```python
from build123d import *

# Parameters (mm, degrees)
SKETCH2_W                 = 304.8
SKETCH2_H                 = 101.6
SKETCH2_R                 = 6.35
SKETCH2_R_2               = 7
BOSS_EXTRUDE1_DEPTH       = 20
SKETCH3_R                 = 3.25
CUT_EXTRUDE1_DEPTH        = 162.883909021
CIRPATTERN1_COUNT         = 4
LPATTERN1_COUNT           = 2
LPATTERN1_PITCH           = 152.4
LPATTERN1_COPY_1_SKETCH_R = 3.25
LPATTERN1_COPY_1_DEPTH    = 162.883909021
LPATTERN1_COPY_2_SKETCH_R = 3.25
LPATTERN1_COPY_2_DEPTH    = 162.883909021
LPATTERN1_COPY_3_SKETCH_R = 3.25
LPATTERN1_COPY_3_DEPTH    = 162.883909021
SKETCH4_W                 = 35.387760229
SKETCH4_H                 = 49.864571232
CUT_EXTRUDE2_DEPTH        = 5


with BuildPart() as part:
    # Sketch2 → Boss-Extrude1 (new body)
    with BuildSketch(Plane(origin=(0, 0, 0), x_dir=(1, 0, 0), z_dir=(0, 1, 0))):
        Rectangle(SKETCH2_W, SKETCH2_H)
        with Locations(Location((0, 0, 0), (0, 0, 270))):
            Circle(SKETCH2_R, mode=Mode.SUBTRACT)
        with Locations(Location((-76.2, 0, 0), (0, 0, 270))):
            Circle(SKETCH2_R_2, mode=Mode.SUBTRACT)
        with Locations(Location((76.2, 0, 0), (0, 0, 270))):
            Circle(SKETCH2_R_2, mode=Mode.SUBTRACT)
    extrude(amount=BOSS_EXTRUDE1_DEPTH)

    # Sketch3 → Cut-Extrude1 (cut, through all)
    with BuildSketch(Plane(origin=(0, 20, 0), x_dir=(1, 0, 0), z_dir=(0, 1, 0))):
        with Locations(Location((-76.2, 19, 0), (0, 0, 270))):
            Circle(SKETCH3_R)
    cut_extrude1 = extrude(amount=-CUT_EXTRUDE1_DEPTH, mode=Mode.SUBTRACT)

    # CirPattern1: Cut-Extrude1 ×4 about axis
    cirpattern1_axis = Axis((-76.2, 0, 0), (0, 1, 0))
    for i in range(1, CIRPATTERN1_COUNT):
        add(cut_extrude1.rotate(cirpattern1_axis, i * 360 / CIRPATTERN1_COUNT), mode=Mode.SUBTRACT)

    # LPattern1: Cut-Extrude1 ×2
    with Locations(*[(i * LPATTERN1_PITCH, 0, 0) for i in range(1, LPATTERN1_COUNT)]):
        add(cut_extrude1, mode=Mode.SUBTRACT)

    # LPattern1 copy 1 sketch → LPattern1 copy 1 (cut, through all)
    with BuildSketch(Plane(origin=(76.2, 20, -76.2), x_dir=(0, 0, -1), z_dir=(0, 1, 0))):
        with Locations(Location((-76.2, 19, 0), (0, 0, 270))):
            Circle(LPATTERN1_COPY_1_SKETCH_R)
    extrude(amount=-LPATTERN1_COPY_1_DEPTH, mode=Mode.SUBTRACT)

    # LPattern1 copy 2 sketch → LPattern1 copy 2 (cut, through all)
    with BuildSketch(Plane(origin=(0, 20, 0), x_dir=(-1, 0, 0), z_dir=(0, 1, 0))):
        with Locations(Location((-76.2, 19, 0), (0, 0, 270))):
            Circle(LPATTERN1_COPY_2_SKETCH_R)
    extrude(amount=-LPATTERN1_COPY_2_DEPTH, mode=Mode.SUBTRACT)

    # LPattern1 copy 3 sketch → LPattern1 copy 3 (cut, through all)
    with BuildSketch(Plane(origin=(76.2, 20, 76.2), x_dir=(0, 0, 1), z_dir=(0, 1, 0))):
        with Locations(Location((-76.2, 19, 0), (0, 0, 270))):
            Circle(LPATTERN1_COPY_3_SKETCH_R)
    extrude(amount=-LPATTERN1_COPY_3_DEPTH, mode=Mode.SUBTRACT)

    # Sketch4 → Cut-Extrude2 (cut)
    with BuildSketch(Plane(origin=(0, 20, 0), x_dir=(1, 0, 0), z_dir=(0, 1, 0))):
        with Locations((-124.178867714, 0)):
            Rectangle(SKETCH4_W, SKETCH4_H)
        with Locations((124.178867714, 0)):
            Rectangle(SKETCH4_W, SKETCH4_H)
    extrude(amount=-CUT_EXTRUDE2_DEPTH, mode=Mode.SUBTRACT)


solid = part.part
```
Work out the finished part from the listing and answer in its coordinate system (mm). A direction names the side the tool comes from. Round coordinates to 2 decimals unless told otherwise and drop trailing zeros. Order: outer loops, then holes, each group sorted by start corner. A loop starts at its lowest first (then second) coordinate and runs counter-clockwise, first axis right, second up.
Q1. Find the intervals of material crossed by line 1 along X through (y, z) = (10.25, 19); line 2 along X through (y, z) = (6.75, 5); line 3 along Y through (x, z) = (122, 0), in increasing order.
Solution:
line 1: x = -152.4 to -79.45, -72.95 to 72.95, 79.45 to 152.4
line 2: x = -152.4 to -81.1, -71.3 to -3.91, 3.91 to 71.3, 81.1 to 152.4
line 3: y = 0 to 15
Q2. A cutting plane is placed at D-D, the plane z = 19. Determine the outline of the cut face in (x, y).
Solution:
outline: (-152.4, 0) - (-79.45, 0) - (-79.45, 20) - (-106.48, 20) - (-106.48, 15) - (-141.87, 15) - (-141.87, 20) - (-152.4, 20) - close; (-72.95, 0) - (72.95, 0) - (72.95, 20) - (-72.95, 20) - close; (79.45, 0) - (152.4, 0) - (152.4, 20) - (141.87, 20) - (141.87, 15) - (106.48, 15) - (106.48, 20) - (79.45, 20) - close
Q3. A cutting plane is placed at C-C, the plane x = 0. Determine the outline of the cut face in (y, z), then the cut area to 3 significant figures.
Solution:
outline: (0, -50.8) - (20, -50.8) - (20, -6.35) - (0, -6.35) - close; (0, 6.35) - (20, 6.35) - (20, 50.8) - (0, 50.8) - close
area: 1,780 mm2
Q4. A cutting plane is placed at B-B, the plane y = 9.25. Count the separate pieces of the cut face and the enclosed holes in it, then the cut area to 3 significant figures.
Solution:
separate pieces: 1
enclosed holes: 11
area: 30,300 mm2
Q5. Given pin 1 Ø4 at (x, z) = (-76.2, 19) entering from -Y; pin 2 Ø10.5 at (x, z) = (76.2, -19) entering from +Y; pin 3 Ø17.5 at (x, z) = (120.5, 0.5) entering from +Y, each flat-ended and moving along its own axis, determine where each tip first touches the part or whether it passes through.
Solution:
pin 1: passes through
pin 2: stops at y = 20
pin 3: stops at y = 15
Q6. A cutting plane is placed at A-A, the plane x = 76.2. Determine the outline of the cut face in (y, z), then the cut area to 3 significant figures.
Solution:
outline: (0, -50.8) - (20, -50.8) - (20, -22.25) - (0, -22.25) - close; (0, -15.75) - (20, -15.75) - (20, -7) - (0, -7) - close; (0, 7) - (20, 7) - (20, 15.75) - (0, 15.75) - close; (0, 22.25) - (20, 22.25) - (20, 50.8) - (0, 50.8) - close
area: 1,490 mm2
Q7. The mould has two halves that part along Z. Classify faces 1 (the flat face through (-2, 10, -50.8)), 2 (the flat face through (-152.4, 10, 1)), 3 (the cylindrical face through (-79.373, 10.14, -19.705)): pulls with the +Z half, pulls with the -Z half, needs draft (parallel to the pull), parting line crosses it, or undercut.
Solution:
face 1: pulls with the -Z half
face 2: needs draft
face 3: undercut
Q8. A tool of negligible diameter and unlimited length cuts with its end or side. For faces 4 (the flat face through (-124, 15, 0)), 5 (the flat face through (-2, 10, 50.8)), from which of +Z, -Z, +X, -X, +Y, -Y can it reach the whole face along a straight path? Write none if from no direction.
Solution:
face 4: +Y
face 5: +Z, +X, -X, +Y, -Y
